Source: CAD feature listing. Evaluate the final solid. Frame: model axes, mm. Face numbers are marked on the shaded views. A direction names the side the tool comes from. Round coordinates to 2 decimals unless told otherwise and drop trailing zeros. Order: outer loops, then holes, each group sorted by start corner. A loop starts at its lowest first (then second) coordinate and runs counter-clockwise, first axis right, second up. Notation, with made-up numbers: (-2.5, 8.25) - (51.5, 8.25) arc R24 ccw to (51.5, 36.25) - close; hole circle Ø10 at (-3.75, 17.25). An arc over 180 degrees is marked (long way). Put each result on its own line as item: value. Start each with the question number.
1) Section A-A on y = 8. Output: boundary loops of the cut face in (x, z), then the cut area to 3 significant figures.
2) Line query: probe 1 along X at (y, z) = (18, -0.05); probe 2 along Y at (x, z) = (-1.2, 0.05). Output: solid intervals per line, ascending. Write a range as [from, to].
3) Contact query for flat-ended pins moving along their axis: P1, Ø2, axis at y = 24.5, z = -1.5, coming from the +X side; P2, Ø1.5, axis at x = -0.5, z = 0, coming from the -Y side. Output: stop coordinate, or through.
4) Access query for the marked faces 1 and 2. Directions: +Z, -Z, +X, -X, +Y, -Y. A direction counts if a zero-diameter tool reaches every point of the face in a straight line with its end or side. Return the directions, or none.
```python
from build123d import *

# Parameters (mm, degrees)
SKETCH1_R           = 1.5
BOSS_EXTRUDE1_DEPTH = 40
SKETCH2_R           = 2.6
BOSS_EXTRUDE2_DEPTH = 1.7
BOSS_EXTRUDE2_TAPER = 32
SKETCH3_W           = 0.5
SKETCH3_H           = 1.758378485
SKETCH3_H_2         = 1.741621515
SKETCH3_W_2         = 1.734727157
SKETCH3_H_3         = 0.5
SKETCH3_W_3         = 1.765272843
CUT_EXTRUDE1_DEPTH  = 0.3


with BuildPart() as part:
    # Sketch1 → Boss-Extrude1 (new body)
    with BuildSketch(Plane(origin=(0, 0, 0), x_dir=(1, 0, 0), z_dir=(0, 1, 0))):
        Circle(SKETCH1_R)
    extrude(amount=BOSS_EXTRUDE1_DEPTH)

    # Sketch2 → Boss-Extrude2 (add)
    with BuildSketch(Plane(origin=(0, 40, 0), x_dir=(1, 0, 0), z_dir=(0, 1, 0))):
        Circle(SKETCH2_R)
    extrude(amount=-BOSS_EXTRUDE2_DEPTH, taper=BOSS_EXTRUDE2_TAPER)

    # Sketch3 → Cut-Extrude1 (cut)
    with BuildSketch(Plane(origin=(0, 40, 0), x_dir=(1, 0, 0), z_dir=(0, 1, 0))):
        with Locations((-0.015272843, 1.120810757)):
            Rectangle(SKETCH3_W, SKETCH3_H)
        with Locations((-0.015272843, -1.129189243)):
            Rectangle(SKETCH3_W, SKETCH3_H_2)
        with Locations((-1.132636421, -0.008378485)):
            Rectangle(SKETCH3_W_2, SKETCH3_H_3)
        with Locations((1.117363579, -0.008378485)):
            Rectangle(SKETCH3_W_3, SKETCH3_H_3)
        with Locations((-0.015272843, -0.008378485)):
            Rectangle(SKETCH3_W, SKETCH3_H_3)
    extrude(amount=-CUT_EXTRUDE1_DEPTH, mode=Mode.SUBTRACT)


solid = part.part
```
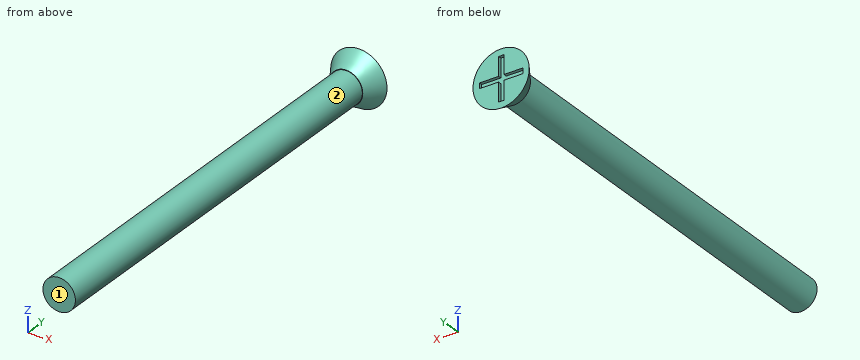
Answer sheet:
1. outline: circle Ø3 at (0, 0)
1. area: 7.07 mm^2
2. probe 1: [-1.5, 1.5]
2. probe 2: [0, 39.7]
3. P1: x = 1.41
3. P2: y = 0
4. face 1: +Z, -Z, +X, -X, -Y
4. face 2: -Y
